Model file for the job. Use its own axes, mm. A direction names the side the tool comes from. Coordinates: 2 decimals unless noted, no trailing zeros. Write each loop counter-clockwise with the first axis right and the second up, starting at its lowest first coordinate (ties: lowest second). Pieces come first, ordered by that corner, then holes.
Q1. Band-saw the part on C-C, the plane x = -4.5. Write the cut outline in (y, z).
Q2. Band-saw the part on B-B, the plane y = 12.5. Write the cut outline in (x, z), plus the area to 3 significant figures.
Q3. Pull direction Z, two halves, no side cores. Call faces 5 (the cylindrical face through (-5, -4, 0)), 6 (the flat face through (4, 19, 6)), 7 (the cylindrical face through (0.466, -4.056, -1.478)): released by +Z, released by -Z, zero draft, split by the parting line, or undercut.
Q4. Drill centre lines: probe 1 along Z at (x, y) = (0.25, 37); probe 2 along X at (y, z) = (13.5, -0.25); probe 3 along Y at (x, z) = (-7.5, -3.25). Where is each one in solid material? Low to high.
Q5. Pin check, flat tips, straight feed: P1, Ø1.6, axis at x = 0.5, z = 0, coming from the -Y side; P2, Ø2, axis at y = 18, z = -2.5, coming from the +X side; P3, Ø5, axis at x = 5.5, y = 1.5, coming from the -Z side; P4, Ø1, axis at x = -7, y = 2, coming from the +Z side. Stop position of each tip, or through.
Q6. Band-saw the part on A-A, the plane z = 5.25. Write the cut outline in (x, y).
Q7. Which spindle directions (+Z, -Z, +X, -X, +Y, -Y) get a long thin tool onto all of the face, cutting with end or side? Do faces 1 (the flat face through (-7.3, 16.5, 0)), 2 (the cylindrical face through (1.98, 21.03, 6.7)), 3 (the flat face through (7, 14, -6)), 4 (the flat face through (0, -4, -3.969)). Say none if no direction does.
Q8. Band-saw the part on D-D, the plane x = 8. Write the cut outline in (y, z), plus the area to 3 significant figures.
from build123d import *

# Parameters (mm, degrees)
SKETCH1_W           = 6.05
SKETCH1_H           = 17
SKETCH1_H_2         = 4
SKETCH1_H_3         = 5
SKETCH1_H_4         = 10
SKETCH1_5_W         = 3
SKETCH1_5_H         = 4
SKETCH1_6_W         = 3
SKETCH1_6_H         = 4
SKETCH2_W           = 8.55
SKETCH2_H           = 2.5
SKETCH2_3_W         = 8.55
SKETCH2_3_H         = 2.5
BOSS_EXTRUDE1_DEPTH = 8
SKETCH4_R           = 1.55
CUT_EXTRUDE1_DEPTH  = 8


with BuildPart() as part:
    # Sketch1 → Revolve4 (revolve)
    with BuildSketch(Plane.XY, mode=Mode.PRIVATE) as revolve4_sk:
        with Locations((-3.025, 31.5)):
            Rectangle(SKETCH1_W, SKETCH1_H)
        with Locations((-3.025, 21)):
            Rectangle(SKETCH1_W, SKETCH1_H_2)
        with Locations((-3.025, 16.5)):
            Rectangle(SKETCH1_W, SKETCH1_H_3)
        with Locations((-3.025, 12)):
            Rectangle(SKETCH1_W, SKETCH1_H_2)
        with Locations((-3.025, 5)):
            Rectangle(SKETCH1_W, SKETCH1_H_4)
    revolve(revolve4_sk.sketch.rotate(Axis((0, 0, 0), (0, 1, 0)), 270), axis=Axis((0, 0, 0), (0, 1, 0)))

    # Sketch1<5> → Revolve5 (revolve)
    with BuildSketch(Plane.XY, mode=Mode.PRIVATE) as revolve5_sk:
        with Locations((-7.55, 21)):
            Rectangle(SKETCH1_5_W, SKETCH1_5_H)
    revolve(revolve5_sk.sketch.rotate(Axis((-1.5, 0, 0), (0, 1, 0)), 180), axis=Axis((-1.5, 0, 0), (0, 1, 0)))

    # Sketch1<6> → Revolve6 (revolve)
    with BuildSketch(Plane.XY, mode=Mode.PRIVATE) as revolve6_sk:
        with Locations((7.55, 12)):
            Rectangle(SKETCH1_6_W, SKETCH1_6_H)
    revolve(revolve6_sk.sketch.rotate(Axis((1.5, 0, 0), (0, 1, 0)), 180), axis=Axis((1.5, 0, 0), (0, 1, 0)))

    # Sketch2 → Revolve7 (revolve)
    with BuildSketch(Plane.XY, mode=Mode.PRIVATE) as revolve7_sk:
        with Locations((-5.775, 17.75)):
            Rectangle(SKETCH2_W, SKETCH2_H)
    revolve(revolve7_sk.sketch.rotate(Axis((-1.5, 19, 0), (0, -1, 0)), 270), axis=Axis((-1.5, 19, 0), (0, -1, 0)))

    # Sketch2<3> → Revolve8 (revolve)
    with BuildSketch(Plane.XY, mode=Mode.PRIVATE) as revolve8_sk:
        with Locations((5.775, 15.25)):
            Rectangle(SKETCH2_3_W, SKETCH2_3_H)
    revolve(revolve8_sk.sketch.rotate(Axis((1.5, 19, 0), (0, -1, 0)), 90), axis=Axis((1.5, 19, 0), (0, -1, 0)))

    # Sketch3 → Boss-Extrude1 (add)
    with BuildSketch(Plane.XZ):
        with BuildLine():
            Line((3.041220715, 3.96875), (-3.041220715, 3.96875))
            ThreePointArc((-3.041220715, 3.96875), (-5, 0), (-3.041220715, -3.96875))
            Line((-3.041220715, -3.96875), (3.041220715, -3.96875))
            ThreePointArc((3.041220715, -3.96875), (4.483642692, -2.212904926), (5, 0))
            ThreePointArc((5, 0), (4.483642692, 2.212904926), (3.041220715, 3.96875))
        make_face()
    extrude(amount=BOSS_EXTRUDE1_DEPTH)

    # Sketch4 → Cut-Extrude1 (cut)
    with BuildSketch(Plane.XZ.offset(8)):
        with Locations(Location((0, 0, 0), (0, 0, 270))):
            Circle(SKETCH4_R)
    extrude(amount=-CUT_EXTRUDE1_DEPTH, mode=Mode.SUBTRACT)


solid = part.part
Answer sheet:
1. outline: (-8, -2.18) - (0, -2.18) - (0, -4.04) - (10, -4.04) - (10, -4.58) - (14, -4.58) - (14, -6.09) - (16.5, -6.09) - (16.5, -8.01) - (19, -8.01) - (19, -6.93) - (23, -6.93) - (23, -4.04) - (40, -4.04) - (40, 4.04) - (23, 4.04) - (23, 6.93) - (19, 6.93) - (19, 8.01) - (16.5, 8.01) - (16.5, 6.09) - (14, 6.09) - (14, 4.58) - (10, 4.58) - (10, 4.04) - (0, 4.04) - (0, 2.18) - (-8, 2.18) - close
2. outline: circle Ø15.1 at (1.5, 0)
2. area: 179 mm2
3. face 5: split by the parting line
3. face 6: zero draft
3. face 7: undercut
4. probe 1: z = -6.04 to 6.04
4. probe 2: x = -6.05 to 9.05
4. probe 3: y = 16.5 to 23
5. P1: stops at y = 0
5. P2: stops at x = 6.92
5. P3: stops at z = -5.25
5. P4: passes through
6. outline: (-8.25, 16.5) - (-5.25, 16.5) - (-5.25, 14) - (-3.93, 14) - (-3.93, 10) - (-3.01, 10) - (-3.01, 0) - (3.01, 0) - (3.01, 10) - (6.93, 10) - (6.93, 14) - (8.25, 14) - (8.25, 16.5) - (5.25, 16.5) - (5.25, 19) - (3.93, 19) - (3.93, 23) - (3.01, 23) - (3.01, 40) - (-3.01, 40) - (-3.01, 23) - (-6.93, 23) - (-6.93, 19) - (-8.25, 19) - close
7. face 1: -X, -Y
7. face 2: +Y
7. face 3: -Y
7. face 4: -Z, +X, -X, -Y
8. outline: (10, -3.84) - (14, -3.84) - (14, -5.55) - (16.5, -5.55) - (16.5, 5.55) - (14, 5.55) - (14, 3.84) - (10, 3.84) - close
8. area: 58.5 mm2
